Build history of the part. All positions in model axes, mm. Coordinates: 2 decimals unless noted, no trailing zeros. Order: outer loops, then holes, each group sorted by start corner. A loop starts at its lowest first (then second) coordinate and runs counter-clockwise, first axis right, second up. Notation, with made-up numbers: M 53,76 L 70,76 A19 ccw 70,92 Z; hole C 67,33.25 d9. An arc over 180 degrees is marked long. Use a Markdown table: item, result. Add a question column.
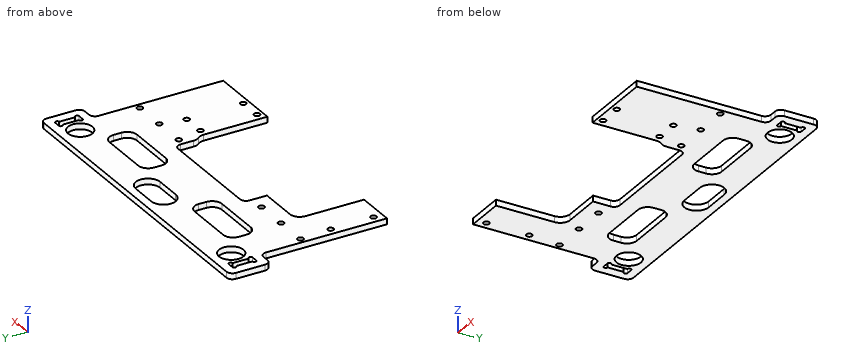
from build123d import *

# Parameters (mm, degrees)
SKETCH_1_W          = 165
SKETCH_1_H          = 51
EXTRUDE_1_DEPTH     = 3
SKETCH_2_R          = 1.5
CUT_EXTRUDE_1_DEPTH = 87.403124943
SKETCH_3_R          = 6.25
SKETCH_3_W          = 3.1
SKETCH_3_H          = 12.2
CUT_EXTRUDE_2_DEPTH = 87.403124943
SKETCH_5_W          = 9.5
SKETCH_5_H          = 30
CUT_EXTRUDE_4_DEPTH = 87.403124943
FILLET_1_R          = 3
SKETCH_6_W          = 20
SKETCH_6_H          = 35
SKETCH_6_W_2        = 38.5
SKETCH_6_H_2        = 37
EXTRUDE_2_DEPTH     = 3
SKETCH_4_R          = 1
CUT_EXTRUDE_3_DEPTH = 104.544676348
SKETCH_8_R          = 1.5
CUT_EXTRUDE_6_DEPTH = 104.544676348
FILLET_2_R          = 5
SKETCH_10_W         = 35
SKETCH_10_H         = 14
CUT_EXTRUDE_8_DEPTH = 104.544676348
FILLET_3_R          = 5
SKETCH_11_W         = 60
SKETCH_11_H         = 12
CUT_EXTRUDE_9_DEPTH = 104.544676348
FILLET_4_R          = 3
FILLET_5_R          = 5
FILLET_6_R          = 5


with BuildPart() as part:
    # 草图1 → 凸台-拉伸1 (new body)
    with BuildSketch(Plane.XY):
        Rectangle(SKETCH_1_W, SKETCH_1_H)
    extrude(amount=EXTRUDE_1_DEPTH)

    # 草图2 → 切除-拉伸1 (cut, through all)
    with BuildSketch(Plane.XY.offset(3)):
        with Locations((-53, -18)):
            Circle(SKETCH_2_R)
        with Locations((-36, -18)):
            Circle(SKETCH_2_R)
        with Locations(Location((36, -18, 0), (0, 0, 180))):
            Circle(SKETCH_2_R)
        with Locations(Location((53, -18, 0), (0, 0, 180))):
            Circle(SKETCH_2_R)
        with Locations((-70, -18)):
            Circle(SKETCH_2_R)
        with Locations(Location((70, -18, 0), (0, 0, 180))):
            Circle(SKETCH_2_R)
    extrude(amount=-CUT_EXTRUDE_1_DEPTH, mode=Mode.SUBTRACT)

    # 草图3 → 切除-拉伸2 (cut, through all)
    with BuildSketch(Plane.XY.offset(3)):
        with Locations((-65.75, 15)):
            Circle(SKETCH_3_R)
        with Locations(Location((65.75, 15, 0), (0, 0, 180))):
            Circle(SKETCH_3_R)
        with BuildLine():
            Line((-6.75, 21.25), (6.75, 21.25))
            ThreePointArc((6.75, 21.25), (13, 15), (6.75, 8.75))
            Line((6.75, 8.75), (-6.75, 8.75))
            ThreePointArc((-6.75, 8.75), (-13, 15), (-6.75, 21.25))
        make_face()
        with Locations((-75.55, 15)):
            Rectangle(SKETCH_3_W, SKETCH_3_H)
        with Locations((75.55, 15)):
            Rectangle(SKETCH_3_W, SKETCH_3_H)
    extrude(amount=-CUT_EXTRUDE_2_DEPTH, mode=Mode.SUBTRACT)

    # 草图5 → 切除-拉伸4 (cut, through all)
    with BuildSketch(Plane(origin=(0, 0, 0), x_dir=(-1, 0, 0), z_dir=(0, 0, -1))):
        with Locations((-77.75, -10.5)):
            Rectangle(SKETCH_5_W, SKETCH_5_H)
        with Locations((77.75, -10.5)):
            Rectangle(SKETCH_5_W, SKETCH_5_H)
    extrude(amount=-CUT_EXTRUDE_4_DEPTH, mode=Mode.SUBTRACT)

    # 圆角1
    fillet_1_edges = [part.edges().sort_by_distance(p)[0] for p in [
        (82.5, 4.5, 1.5),
        (73, 4.5, 1.5),
        (-73, 4.5, 1.5),
        (-82.5, 4.5, 1.5),
        (-82.5, 25.5, 1.5),
        (82.5, 25.5, 1.5),
    ]]
    fillet(fillet_1_edges, radius=FILLET_1_R)

    # 草图6 → 凸台-拉伸2 (add)
    with BuildSketch(Plane(origin=(0, 0, 0), x_dir=(-1, 0, 0), z_dir=(0, 0, -1))):
        with Locations((63, -43)):
            Rectangle(SKETCH_6_W, SKETCH_6_H)
        with Locations((-53.75, -44)):
            Rectangle(SKETCH_6_W_2, SKETCH_6_H_2)
    extrude(amount=-EXTRUDE_2_DEPTH)

    # 草图4 → 切除-拉伸3 (cut, through all)
    with BuildSketch(Plane.XY.offset(3)):
        with Locations((-74, 20.1)):
            Circle(SKETCH_4_R)
        with Locations((-74, 9.9)):
            Circle(SKETCH_4_R)
        with Locations((-77.1, 9.9)):
            Circle(SKETCH_4_R)
        with Locations((-77.1, 20.1)):
            Circle(SKETCH_4_R)
        with Locations((77.1, 20.1)):
            Circle(SKETCH_4_R)
        with Locations((77.1, 9.9)):
            Circle(SKETCH_4_R)
        with Locations((74, 9.9)):
            Circle(SKETCH_4_R)
        with Locations((74, 20.1)):
            Circle(SKETCH_4_R)
    extrude(amount=-CUT_EXTRUDE_3_DEPTH, mode=Mode.SUBTRACT)

    # 草图8 → 切除-拉伸6 (cut, through all)
    with BuildSketch(Plane.XY.offset(3)):
        with Locations((-69, -56)):
            Circle(SKETCH_8_R)
        with Locations((-69, -34)):
            Circle(SKETCH_8_R)
        with Locations((38.5, -30.5)):
            Circle(SKETCH_8_R)
        with Locations((38.5, -59.5)):
            Circle(SKETCH_8_R)
        with Locations((50.5, -59.5)):
            Circle(SKETCH_8_R)
        with Locations((50.5, -30.5)):
            Circle(SKETCH_8_R)
    extrude(amount=-CUT_EXTRUDE_6_DEPTH, mode=Mode.SUBTRACT)

    # 圆角2
    fillet_2_edges = [part.edges().sort_by_distance(p)[0] for p in [
        (-53, -25.5, 1.5),
    ]]
    fillet(fillet_2_edges, radius=FILLET_2_R)

    # 草图10 → 切除-拉伸8 (cut, through all)
    with BuildSketch(Plane.XY.offset(3)):
        with Locations((37, 2.5)):
            Rectangle(SKETCH_10_W, SKETCH_10_H)
        with Locations((-37, 2.5)):
            Rectangle(SKETCH_10_W, SKETCH_10_H)
    extrude(amount=-CUT_EXTRUDE_8_DEPTH, mode=Mode.SUBTRACT)

    # 圆角3
    fillet_3_edges = [part.edges().sort_by_distance(p)[0] for p in [
        (-19.5, 9.5, 1.5),
        (-19.5, -4.5, 1.5),
        (-54.5, -4.5, 1.5),
        (-54.5, 9.5, 1.5),
        (54.5, 9.5, 1.5),
        (54.5, -4.5, 1.5),
        (19.5, -4.5, 1.5),
        (19.5, 9.5, 1.5),
    ]]
    fillet(fillet_3_edges, radius=FILLET_3_R)

    # 草图11 → 切除-拉伸9 (cut, through all)
    with BuildSketch(Plane.XY.offset(3)):
        with Locations((2, -19.5)):
            Rectangle(SKETCH_11_W, SKETCH_11_H)
    extrude(amount=-CUT_EXTRUDE_9_DEPTH, mode=Mode.SUBTRACT)

    # 圆角4
    fillet_4_edges = [part.edges().sort_by_distance(p)[0] for p in [
        (-28, -13.5, 1.5),
        (32, -13.5, 1.5),
    ]]
    fillet(fillet_4_edges, radius=FILLET_4_R)

    # 圆角5
    # the kernel refuses this fillet: 5 mm, written as the material it adds along each edge
    with BuildSketch(Plane(origin=(34.5, -25.5, 0), x_dir=(-1, 0, 0), z_dir=(0, 0, 1))) as fillet_5_piece_1:
        with BuildLine():
            CenterArc((5, 4.330127019), FILLET_5_R, 180, 60)
            Line((0, 4.330127019), (-0.1, 4.330127019))
            Line((-0.1, 4.330127019), (-0.1, 0))
            Line((-0.1, 0), (0, -0.1))
            ThreePointArc((0, -0.1), (1.25, -0.1), (2.45, -0.08660254))
            Line((2.45, -0.08660254), (2.5, 0))
        make_face()
    extrude(amount=3)

    # 圆角6
    fillet_6_edges = [part.edges().sort_by_distance(p)[0] for p in [
        (32, -25.5, 1.5),
    ]]
    fillet(fillet_6_edges, radius=FILLET_6_R)


solid = part.part
(1) Slice it at B-B on y = -2.5. Give the cut face in (x, z).
(2) Slice it at C-C on y = -44.5. Give the cut face in (x, z), and give its area (4 significant figures).
(3) Drill centre lines: line 1 along X through (y, z) = (14.5, 1.1); line 2 along Y through (x, z) = (38.5, 1.75); line 3 along X through (y, z) = (5.5, 1.9). Where is each one in solid material? Low to high. Write a range as from..to.
(4) Slice it at D-D on x = -65.75. Give the cut face in (y, z), and give its area (4 significant figures).
(5) Drop flat-ended pins along their axis: P1, Ø0.9, axis at y = -20.5, z = 1, coming from the -X side; P2, Ø1.5, axis at x = -77.5, z = 1, coming from the -Y side. Give the stop position or say it passes through.
(6) Slice it at A-A on x = -36. Give the cut face in (y, z), and give its area (3 significant figures).
Solutions:
| question | item | result |
|---|---|---|
| 1 | outline | M -73,0 L -53.5,0 L -53.5,3 L -73,3 Z; M -20.5,0 L 20.5,0 L 20.5,3 L -20.5,3 Z; M 53.5,0 L 73,0 L 73,3 L 53.5,3 Z |
| 2 | outline | M -73,0 L -53,0 L -53,3 L -73,3 Z; M 34.5,0 L 73,0 L 73,3 L 34.5,3 Z |
| 2 | area | 175.5 mm² |
| 3 | line 1 | -82.5..-77.1, -74..-71.98, -59.52..-12.98, 12.98..59.52, 71.98..74, 77.1..82.5 |
| 3 | line 2 | -62.5..-61, -58..-32, -29..-4.5, 9.5..25.5 |
| 3 | line 3 | -81.74..-54.4, -19.6..19.6, 54.4..81.74 |
| 4 | outline | M -60.5,0 L 8.75,0 L 8.75,3 L -60.5,3 Z; M 21.25,0 L 25.5,0 L 25.5,3 L 21.25,3 Z |
| 4 | area | 220.5 mm² |
| 5 | P1 | x = -73 |
| 5 | P2 | y = 4.5 |
| 6 | outline | M -25.5,0 L -19.5,0 L -19.5,3 L -25.5,3 Z; M -16.5,0 L -4.5,0 L -4.5,3 L -16.5,3 Z; M 9.5,0 L 25.5,0 L 25.5,3 L 9.5,3 Z |
| 6 | area | 102 mm² |
